Part model, mm, in its own coordinate system. A direction names the side the tool comes from. Give positions to 0.01 mm unless a question says otherwise; leave off trailing zeros. Order: outer loops, then holes, each group sorted by start corner. A loop starts at its lowest first (then second) coordinate and runs counter-clockwise, first axis right, second up.
1. Drop flat-ended pins along their axis: pin 1 Ø3 at (y, z) = (-0.5, 8.5) entering from +X; pin 2 Ø1 at (y, z) = (-1.5, 17.5) entering from -X; pin 3 Ø6 at (x, y) = (-6, 1) entering from +Z. Give the stop position or say it passes through.
2. Which spindle directions (+Z, -Z, +X, -X, +Y, -Y) get a long thin tool onto all of the face, cutting with end or side? Do faces 1 (the flat face through (10, -5, 26.5)), 2 (the flat face through (-14, 0, 23)), 3 (the flat face through (3, -1, 31.5)), 4 (the flat face through (-14, 0, 21)). Say none if no direction does.
3. Slice it at D-D on y = 3.5. List the corners of the cut face in (x, z).
4. Slice it at A-A on y = -5. List the corners of the cut face in (x, z), and give its area (3 significant figures).
5. Slice it at C-C on z = 28. List the corners of the cut face in (x, y).
6. Slice it at B-B on x = 13. List the corners of the cut face in (y, z), and give its area (3 significant figures).
7. Probe line 1 (X direction, y = 5.25, z = 14); line 2 (Z direction, x = 14.5, y = 3.75); line 3 (Z direction, x = 6.5, y = -3.5). List the from-to ranges inside material, lowest first.
from build123d import *

# Parameters (mm, degrees)
F0_W     = 22.5
F0_H     = 12
F1_DEPTH = 21
F2_W     = 5
F2_H     = 12
F2_R     = 4
F2_R_2   = 2
F3_DEPTH = 2
F4_DEPTH = 5.5
F5_DEPTH = 9.5
F6_DEPTH = 10.5
F7_DEPTH = 14.5


with BuildPart() as f1:
    # F0 (on Top) → F1 (new body)
    with BuildSketch(Plane.XY):
        Rectangle(F0_W, F0_H)
    extrude(amount=F1_DEPTH)

    # F2 (on face) → F3 (join)
    with BuildSketch(Plane.XY.offset(21)):
        with BuildLine():
            Line((11.25, 6), (5.25, 6))
            ThreePointArc((5.25, 6), (9.4926406871, 4.2426406871), (11.25, 0))
            Line((11.25, 0), (11.25, 6))
        make_face()
        with Locations((-13.75, 0)):
            Rectangle(F2_W, F2_H)
        Polygon((16.25, 6), (11.25, 6), (11.25, 0), (11.25, -6), (16.25, -6), align=None)
        with BuildLine():
            Line((11.25, -6), (11.25, 0))
            ThreePointArc((11.25, 0), (9.4926406871, -4.2426406871), (5.25, -6))
            Line((5.25, -6), (11.25, -6))
        make_face()
        with BuildLine():
            ThreePointArc((11.25, 0), (9.4926406871, 4.2426406871), (5.25, 6))
            ThreePointArc((5.25, 6), (-0.75, 0), (5.25, -6))
            ThreePointArc((5.25, -6), (9.4926406871, -4.2426406871), (11.25, 0))
        make_face()
        with Locations((5.25, 0)):
            Circle(F2_R, mode=Mode.SUBTRACT)
        with Locations((5.25, 0)):
            Circle(F2_R)
        with Locations((5.25, 0)):
            Circle(F2_R_2, mode=Mode.SUBTRACT)
        with BuildLine():
            Line((5.25, 6), (-11.25, 6))
            Line((-11.25, 6), (-11.25, -6))
            Line((-11.25, -6), (5.25, -6))
            ThreePointArc((5.25, -6), (-0.75, 0), (5.25, 6))
        make_face()
    extrude(amount=F3_DEPTH)

    # F2 (on face) → F4 (join)
    with BuildSketch(Plane.XY.offset(21)):
        with BuildLine():
            Line((5.25, 6), (-11.25, 6))
            Line((-11.25, 6), (-11.25, -6))
            Line((-11.25, -6), (5.25, -6))
            ThreePointArc((5.25, -6), (-0.75, 0), (5.25, 6))
        make_face()
        with BuildLine():
            ThreePointArc((11.25, 0), (9.4926406871, 4.2426406871), (5.25, 6))
            ThreePointArc((5.25, 6), (-0.75, 0), (5.25, -6))
            ThreePointArc((5.25, -6), (9.4926406871, -4.2426406871), (11.25, 0))
        make_face()
        with Locations((5.25, 0)):
            Circle(F2_R, mode=Mode.SUBTRACT)
        with Locations((5.25, 0)):
            Circle(F2_R)
        with Locations((5.25, 0)):
            Circle(F2_R_2, mode=Mode.SUBTRACT)
        with BuildLine():
            Line((11.25, -6), (11.25, 0))
            ThreePointArc((11.25, 0), (9.4926406871, -4.2426406871), (5.25, -6))
            Line((5.25, -6), (11.25, -6))
        make_face()
        with BuildLine():
            Line((11.25, 6), (5.25, 6))
            ThreePointArc((5.25, 6), (9.4926406871, 4.2426406871), (11.25, 0))
            Line((11.25, 0), (11.25, 6))
        make_face()
    extrude(amount=F4_DEPTH)

    # F2 (on face) → F5 (join)
    with BuildSketch(Plane.XY.offset(21)):
        with BuildLine():
            ThreePointArc((11.25, 0), (9.4926406871, 4.2426406871), (5.25, 6))
            ThreePointArc((5.25, 6), (-0.75, 0), (5.25, -6))
            ThreePointArc((5.25, -6), (9.4926406871, -4.2426406871), (11.25, 0))
        make_face()
        with Locations((5.25, 0)):
            Circle(F2_R, mode=Mode.SUBTRACT)
        with Locations((5.25, 0)):
            Circle(F2_R)
        with Locations((5.25, 0)):
            Circle(F2_R_2, mode=Mode.SUBTRACT)
    extrude(amount=F5_DEPTH)

    # F2 (on face) → F6 (join)
    with BuildSketch(Plane.XY.offset(21)):
        with Locations((5.25, 0)):
            Circle(F2_R)
        with Locations((5.25, 0)):
            Circle(F2_R_2, mode=Mode.SUBTRACT)
    extrude(amount=F6_DEPTH)

    # F2 (on face) → F7 (join)
    with BuildSketch(Plane.XY.offset(21)):
        with Locations((5.25, 0)):
            Circle(F2_R_2)
    extrude(amount=F7_DEPTH)


solid = f1.part
Data:
1. pin 1: stops at x = 11.25
1. pin 2: stops at x = -11.25
1. pin 3: stops at z = 26.5
2. face 1: +Z, +X, -Y
2. face 2: +Z, -X, +Y, -Y
2. face 3: +Z
2. face 4: -Z, -X, +Y, -Y
3. outline: (-16.25, 21) - (-11.25, 21) - (-11.25, 0) - (11.25, 0) - (11.25, 21) - (16.25, 21) - (16.25, 23) - (11.25, 23) - (11.25, 26.5) - (10.12, 26.5) - (10.12, 30.5) - (7.19, 30.5) - (7.19, 31.5) - (3.31, 31.5) - (3.31, 30.5) - (0.38, 30.5) - (0.38, 26.5) - (-11.25, 26.5) - (-11.25, 23) - (-16.25, 23) - close
4. outline: (-16.25, 21) - (-11.25, 21) - (-11.25, 0) - (11.25, 0) - (11.25, 21) - (16.25, 21) - (16.25, 23) - (11.25, 23) - (11.25, 26.5) - (8.57, 26.5) - (8.57, 30.5) - (1.93, 30.5) - (1.93, 26.5) - (-11.25, 26.5) - (-11.25, 23) - (-16.25, 23) - close
4. area: 643 mm2
5. outline: circle Ø12 at (5.25, 0)
6. outline: (-6, 21) - (6, 21) - (6, 23) - (-6, 23) - close
6. area: 24.0 mm2
7. line 1: x = -11.25 to 11.25
7. line 2: z = 21 to 23
7. line 3: z = 0 to 31.5
